Can you work these out from the model? Positions are in its coordinate system, mm. A direction names the side the tool comes from. Give positions to 0.01 mm unless a question says otherwise; leave off trailing zeros. Write each loop counter-clockwise with the first axis right and the second up, starting at its lowest first coordinate (ties: lowest second). Pieces come first, ordered by that corner, then holes. Notation, with made-up numbers: M 0,-22.75 L 28,-22.75 A33 ccw 28,8.25 Z; hole C 69,42.25 d10. An arc over 180 degrees is marked long. Use CSV: the item, a comma, the result in double quotes. Start each with the question number.
from build123d import *

# Parameters (mm, degrees)
F2_R     = 2.65
F3_DEPTH = 25
F4_R     = 7.429877
F5_R     = 5
F6_R     = 1


with BuildPart() as f1:
    # F0 (on Front) → F1 (revolve)
    with BuildSketch(Plane.XZ):
        with BuildLine():
            Line((0, 25), (0, 0))
            Line((0, 0), (30, 0))
            Line((30, 0), (30, 5))
            Line((30, 5), (13.847623, 5))
            Line((13.847623, 5), (7.389601, 8.067148))
            Line((7.389601, 8.067148), (7.389601, 14.918145))
            ThreePointArc((7.389601, 14.918145), (12.323801, 22.908607), (10.301951, 32.079535))
            Line((10.301951, 32.079535), (0, 32.079535))
            Line((0, 32.079535), (0, 25))
        make_face()
    revolve(axis=Axis((0, 0, 12.5), (0, 0, 1)))

    # F2 (on face) → F3 (cut)
    with BuildSketch(Plane(origin=(0, 0, 0), x_dir=(1, 0, 0), z_dir=(0, 0, -1))):
        with Locations((0, 23.9)):
            Circle(F2_R)
        with Locations((23.9, 0)):
            Circle(F2_R)
        with Locations((0, -23.9)):
            Circle(F2_R)
        with Locations((-23.9, 0)):
            Circle(F2_R)
    extrude(amount=-F3_DEPTH, mode=Mode.SUBTRACT)

    # F4
    f4_edges = [f1.edges().sort_by_distance(p)[0] for p in [
        (-7.389601, 0, 14.918145),
    ]]
    fillet(f4_edges, radius=F4_R)

    # F5
    f5_edges = [f1.edges().sort_by_distance(p)[0] for p in [
        (-7.389601, 0, 8.067148),
        (-13.847623, 0, 5),
    ]]
    fillet(f5_edges, radius=F5_R)

    # F6
    f6_edges = [f1.edges().sort_by_distance(p)[0] for p in [
        (-10.301951, 0, 32.079535),
    ]]
    fillet(f6_edges, radius=F6_R)


solid = f1.part
(1) Thinking about a two-plate mould opening in X: for faces 1 (the face through (1.425, -26.134, 2.465)), 2 (the face through (-1.602, -7.214, 11.454)), 3 (the face through (0, 0, 0)), which applies, released by +X, released by -X, zero draft, split by the parting line, or undercut?
(2) Which directions (+Z, -Z, +X, -X, +Y, -Y) give clear straight access to the entire face, cutting with the end or side of a thin tool? Please do faces 4 (the face through (21.253, -0.117, 2.465)), 5 (the face through (6, 14, 5)).
(3) Will these pins go through, and if not, where does the flat tip stop? pin 1 Ø8 at (x, z) = (0, 19.5) entering from -Y; pin 2 Ø6 at (x, y) = (23.9, 0) entering from +Z; pin 3 Ø12 at (y, z) = (21.5, 20.5) entering from -X; pin 4 Ø1.5 at (y, z) = (11, 20.5) entering from +X.
(4) I want a section at C-C (x = 0). State how many separate pieces and enclosed holes the cut face has, and give its area (3 significant figures).
(5) I want a section at D-D (y = 18.5). Write out the boundary of the cut face in (x, z), and give its area (3 significant figures).
(6) Please list where these lines run through material, in increasing order: L1, parallel to Y at x = 0, z = 2.45; L2, parallel to Y at x = 23, z = 1; L3, parallel to Y at x = 23.9, z = 1.5. Write a range as [from, to].
(7) I want a section at A-A (x = 23.9). Write out the boundary of the cut face in (y, z).
Geometry results:
1,face 1,"undercut"
1,face 2,"split by the parting line"
1,face 3,"zero draft"
2,face 4,"+Z, -Z"
2,face 5,"+Z"
3,pin 1,"stops at y = -12.41"
3,pin 2,"stops at z = 5"
3,pin 3,"passes through"
3,pin 4,"stops at x = 5.68"
4,separate pieces,"3"
4,enclosed holes,"0"
4,area,"807 mm2"
5,outline,"M -23.62,0 L 23.62,0 L 23.62,5 L -23.62,5 Z"
5,area,"236 mm2"
6,L1,"y = [-30, -26.55], [-21.25, 21.25], [26.55, 30]"
6,L2,"y = [-19.26, -2.49], [2.49, 19.26]"
6,L3,"y = [-18.13, -2.65], [2.65, 18.13]"
7,outline,"M -18.13,0 L -2.65,0 L -2.65,5 L -18.13,5 Z; M 2.65,0 L 18.13,0 L 18.13,5 L 2.65,5 Z"
